The drawing under review shows one solid part. Ordinate dimensions are in mm from its lowest x, y, z. Round coordinates to 2 decimals unless told otherwise and drop trailing zeros. Loops run counter-clockwise (first coordinate to the right, second up) from the corner with the lowest first, then second, coordinate; pieces in that order, holes last. Notation, with made-up numbers: (73, 69.25) -> (117, 69.25) arc R33 cw to (117, 99.25) -> close; hole circle Ø2 at (37, 47). An arc over 180 degrees is marked (long way). Use a Markdown table: item, result. Add a question column.
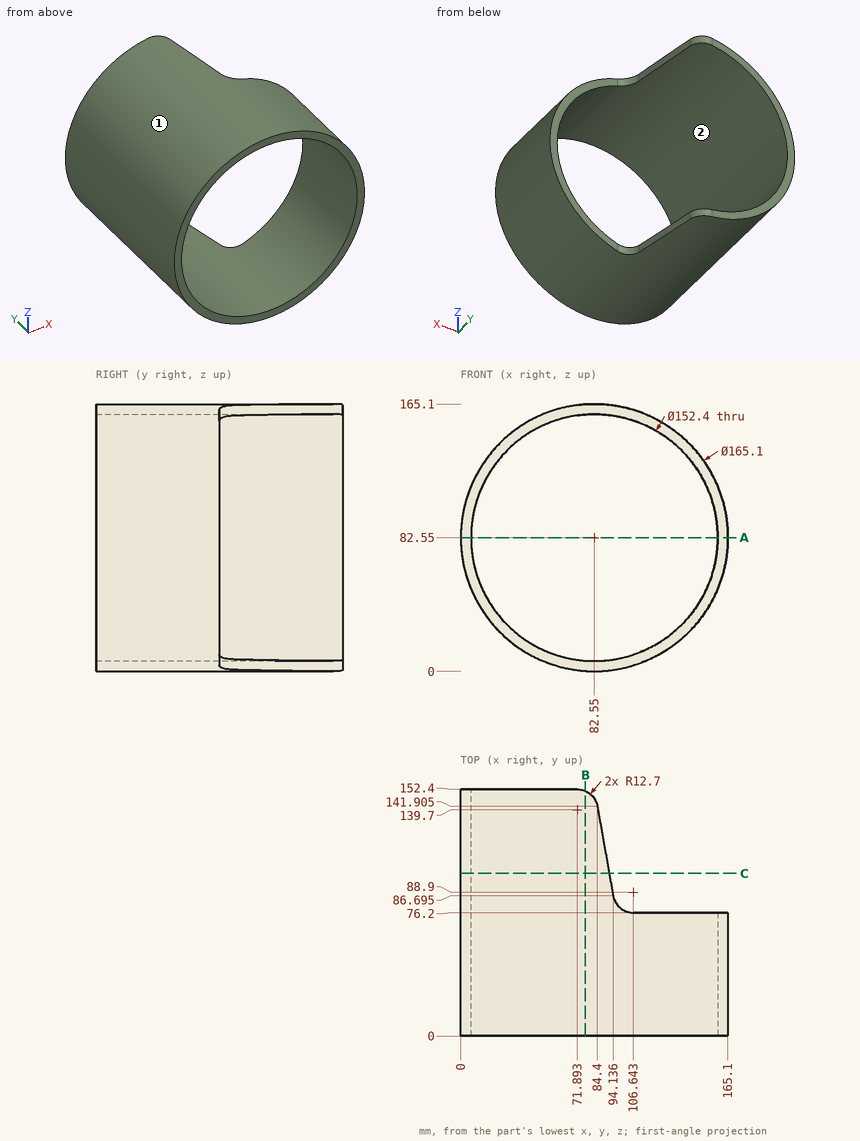
1. Consider section B-B on x = 77. State the section outline as (y, z) points, plus the area to 3 significant figures.
2. To check wall thickness, follow probe 1 along Z at (x, y) = (82.55, 42); probe 2 along Y at (x, z) = (156, 51.5); probe 3 along Z at (x, y) = (140, 74.5). State the ranges of each line that lie inside material, in increasing order. Write a range as from..to.
3. Mouldability with a two-part tool opening along Z and no side actions: class the marked faces 1 and 2 as +Z half, -Z half, draft (parallel to the pull), parting line (faces both ways), or undercut.
4. Consider section A-A on z = 82.55. State the section outline as (x, y) points.
5. Consider section C-C on y = 100.5. State the section outline as (x, z) points.
6. Insertion check: P1, Ø8, axis at x = 42.5, y = 17, coming from the +Z side; P2, Ø1, axis at x = 102.5, y = 75, coming from the -Z side; P3, Ø12, axis at x = 140, z = 147.5, coming from the +Y side. Each pin has a flat end and moves straight along its axis. Give the tip position at first contact, or say it passes through.
Verdict:
| question | item | result |
|---|---|---|
| 1 | outline | (0, 0.19) -> (151.33, 0.19) -> (151.33, 6.55) -> (0, 6.55) -> close; (0, 158.55) -> (151.33, 158.55) -> (151.33, 164.91) -> (0, 164.91) -> close |
| 1 | area | 1,930 mm² |
| 2 | probe 1 | z = 0..6.35, 158.75..165.1 |
| 2 | probe 2 | y = 0..76.2 |
| 2 | probe 3 | z = 23.27..32.49, 132.61..141.83 |
| 3 | face 1 | parting line |
| 3 | face 2 | undercut |
| 4 | outline | (0, 0) -> (6.35, 0) -> (6.35, 152.4) -> (0, 152.4) -> close; (158.75, 0) -> (165.1, 0) -> (165.1, 76.2) -> (158.75, 76.2) -> close |
| 5 | outline | (91.7, 0.51) -> (91.7, 6.9) arc R76.2 cw (long way) to (91.7, 158.2) -> (91.7, 164.59) arc R82.55 ccw (long way) to start |
| 6 | P1 | stops at z = 156.81 |
| 6 | P2 | stops at z = 2.32 |
| 6 | P3 | stops at y = 76.2 |
